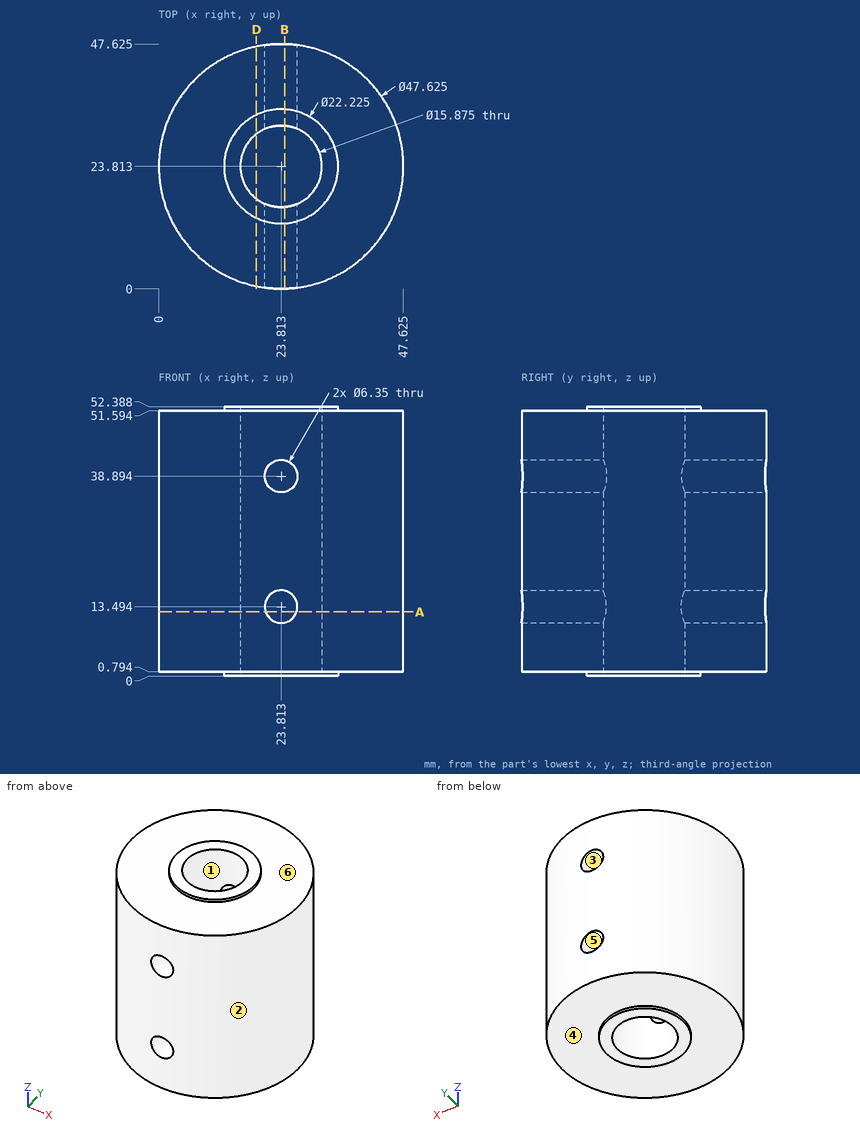
For this review, use the dimensioned drawing (mm, ordinates from the lowest corner) and the shaded views. A direction names the side the tool comes from. Round coordinates to 2 decimals unless told otherwise and drop trailing zeros. Write each loop counter-clockwise with the first axis right and the second up, starting at its lowest first coordinate (ties: lowest second). Pieces come first, ordered by that corner, then holes. Notation, with made-up numbers: (35.5, 45) - (88.5, 45) arc R23 cw to (88.5, 80) - close; hole circle Ø3 at (6, -24). An arc over 180 degrees is marked (long way). One line per item, written item: value. Start each with the question number.
1. Clearance check with flat-ended pins moving along their axes: P1, Ø12, axis at x = 39, z = 31.5, coming from the +Y side; P2, Ø4, axis at x = 27, z = 31, coming from the +Y side (1 decimal); P3, Ø4, axis at x = 32, z = 33, coming from the -Y side. State where each tip first meets the part, or that it passes through.
2. To check wall thickness, follow L1, parallel to Z at x = 44.5, y = 34.5; L2, parallel to X at y = 23.5, z = 5; L3, parallel to X at y = 30, z = 20.5 (1 decimal). State the ranges of each line that lie inside material, in increasing order. Write a range as from..to.
3. Consider section D-D on x = 19. Write out the cut boundary in (y, z) (1 decimal), and give its area (3 significant figures).
4. The part is to be moulded in two halves that separate along Y. For the marked faces 1, 2 and 3, say which applies: released by +Y, released by -Y, zero draft, split by the parting line, or undercut.
5. Machinability: for the marked faces 4, 5 and 6, which of the approach directions +Z, -Z, +X, -X, +Y, -Y give a long, thin tool a straight path to every point of the face, cutting with its end or side? Answer none if there is none.
6. Consider section A-A on z = 12.5. Write out the cut boundary in (x, y) (1 decimal).
7. Consider section B-B on x = 24.5. State how many separate pieces and enclosed holes the cut face has, and give its area (3 significant figures).
Checks:
1. P1: stops at y = 45.78
1. P2: stops at y = 47.6
1. P3: stops at y = 0.82
2. L1: z = 0.79..51.59
2. L2: x = 0..15.88, 31.74..47.62
2. L3: x = 0.8..18.8, 28.8..46.8
3. outline: (0.5, 0.8) - (13.8, 0.8) - (13.8, 0) - (17.5, 0) - (17.5, 52.4) - (13.8, 52.4) - (13.8, 51.6) - (0.5, 51.6) - close; (30.1, 0) - (33.8, 0) - (33.8, 0.8) - (47.1, 0.8) - (47.1, 51.6) - (33.8, 51.6) - (33.8, 52.4) - (30.1, 52.4) - close
3. area: 1,740 mm^2
4. face 1: undercut
4. face 2: split by the parting line
4. face 3: zero draft
5. face 4: -Z
5. face 5: +Y, -Y
5. face 6: +Z
6. outline: (20.8, 0.2) - (20.8, 16.5) arc R7.9 cw to (20.8, 31.2) - (20.8, 47.4) arc R23.8 ccw to start; (26.8, 0.2) arc R23.8 ccw to (26.8, 47.4) - (26.8, 31.2) arc R7.9 cw to (26.8, 16.5) - close
7. separate pieces: 6
7. enclosed holes: 0
7. area: 1,230 mm^2
